```python
from build123d import *

# Parameters (mm, degrees)
CHAMFER1_SIZE = 0.25
FILLET1_R     = 0.4


with BuildPart() as part:
    # Sketch1 → Revolve1 (revolve)
    with BuildSketch(Plane.XY):
        Polygon((0, 0), (0, 1.735), (-22, 1.735), (-22, 4.95), (-28, 4.95), (-28, 0), align=None)
    revolve(axis=Axis((0, 0, 0), (-1, 0, 0)))

    # Chamfer1
    chamfer1_edges = [part.edges().sort_by_distance(p)[0] for p in [
        (0, -1.735, 0),
        (-22, -4.95, 0),
        (-28, -4.95, 0),
    ]]
    chamfer(chamfer1_edges, length=CHAMFER1_SIZE)

    # Fillet1
    fillet1_edges = [part.edges().sort_by_distance(p)[0] for p in [
        (-22, -1.735, 0),
    ]]
    fillet(fillet1_edges, radius=FILLET1_R)


solid = part.part
```
Source: CAD feature listing. Evaluate the final solid. Frame: model axes, mm. A direction names the side the tool comes from. Give positions to 0.01 mm unless a question says otherwise; leave off trailing zeros. Loops run counter-clockwise (first coordinate to the right, second up) from the corner with the lowest first, then second, coordinate; pieces in that order, holes last. Notation, with made-up numbers: (72, 89) -> (114, 89) arc R20 cw to (114, 110) -> close; hole circle Ø7 at (-5.5, -15.5). An arc over 180 degrees is marked (long way). Put each result on its own line as item: value. Start each with the question number.
1) Cut plane C-C (x = -2). Return loops of the section in (y, z) (3 decimals), then the cut area to 3 significant figures.
2) Material intervals for probe 1 along X at (y, z) = (-1.25, -3.75); probe 2 along X at (y, z) = (1.5, -0.5); probe 3 along Z at (x, y) = (-16, -0.25), sorted ascending.
3) Cut plane A-A (y = 0). Return loops of the section in (x, z) (3 decimals).
4) Reachability of faces 1 (the face through (-11.074, 1.655, -0.521)), 2 (the face through (-25.04, 4.72, -1.49)) from +Z, -Z, +X, -X, +Y, -Y: full face, straight path, thin tool, end or side. Return the list, or none.
5) Contact query for flat-ended pins moving along their axis: P1, Ø3, axis at x = -6.5, y = 1.5, coming from the -Z side (3 decimals); P2, Ø3, axis at y = 4, z = 3.5, coming from the +X side; P3, Ø3, axis at x = -14.5, y = 2.5, coming from the +Z side. Output: stop coordinate, or through.
Results are:
1. outline: circle Ø3.47 at (0, 0)
1. area: 9.46 mm2
2. probe 1: x = -28 to -22
2. probe 2: x = -28 to -0.1
2. probe 3: z = -1.72 to 1.72
3. outline: (-28, -4.7) -> (-27.75, -4.95) -> (-22.25, -4.95) -> (-22, -4.7) -> (-22, -2.135) arc R0.4 cw to (-21.6, -1.735) -> (-0.25, -1.735) -> (0, -1.485) -> (0, 1.485) -> (-0.25, 1.735) -> (-21.6, 1.735) arc R0.4 cw to (-22, 2.135) -> (-22, 4.7) -> (-22.25, 4.95) -> (-27.75, 4.95) -> (-28, 4.7) -> close
4. face 1: +X
4. face 2: +X, -X
5. P1: stops at z = -1.735
5. P2: stops at x = -22
5. P3: stops at z = 1.42
